```python
from build123d import *

# Parameters (mm, degrees)
BOSS_EXTRUDE1_DEPTH = 15
SKETCH2_R           = 1.7
SKETCH2_R_2         = 1.35
CUT_EXTRUDE1_DEPTH  = 59.066473529
CUT_EXTRUDE2_DEPTH  = 1


with BuildPart() as part:
    # Sketch1 → Boss-Extrude1 (new body)
    with BuildSketch(Plane.XY):
        with BuildLine():
            Line((0, 0), (35, 0))
            ThreePointArc((35, 0), (43.574008742, 1.66873563), (50.896306384, 6.431325448))
            ThreePointArc((50.896306384, 6.431325448), (52.409115124, 10), (50.896306384, 13.568674552))
            ThreePointArc((50.896306384, 13.568674552), (43.574008742, 18.33126437), (35, 20))
            Line((35, 20), (0, 20))
            Line((0, 20), (0, 17))
            Line((0, 17), (35.015119776, 17))
            ThreePointArc((35.015119776, 17), (42.445641677, 15.557658707), (48.796934125, 11.440124447))
            ThreePointArc((48.796934125, 11.440124447), (49.409115124, 10), (48.796934125, 8.559875553))
            ThreePointArc((48.796934125, 8.559875553), (42.445641677, 4.442341293), (35.015119776, 3))
            Line((35.015119776, 3), (0, 3))
            Line((0, 3), (0, 0))
        make_face()
    extrude(amount=BOSS_EXTRUDE1_DEPTH)

    # Sketch2 → Cut-Extrude1 (cut, through all)
    with BuildSketch(Plane(origin=(0, 20, 0), x_dir=(1, 0, 0), z_dir=(0, 1, 0))):
        with Locations(Location((5, -7.5, 0), (0, 0, 270))):
            Circle(SKETCH2_R)
        with Locations(Location((13.5, -7.5, 0), (0, 0, 270))):
            Circle(SKETCH2_R_2)
        with Locations(Location((31.5, -7.5, 0), (0, 0, 270))):
            Circle(SKETCH2_R_2)
    extrude(amount=-CUT_EXTRUDE1_DEPTH, mode=Mode.SUBTRACT)

    # Sketch3 → Cut-Extrude2 (cut)
    with BuildSketch(Plane.XZ):
        Polygon((5, 10.848631561), (2.1, 9.174315781), (2.1, 5.825684219), (5, 4.151368439), (7.9, 5.825684219), (7.9, 9.174315781), align=None)
    extrude(amount=-CUT_EXTRUDE2_DEPTH, mode=Mode.SUBTRACT)


solid = part.part
```
CAD build for the part. Positions are in the model's coordinates, mm. A direction names the side the tool comes from. Coordinates: 2 decimals unless noted, no trailing zeros. Order: outer loops, then holes, each group sorted by start corner. A loop starts at its lowest first (then second) coordinate and runs counter-clockwise, first axis right, second up. Notation, with made-up numbers: (42.5, 38) - (57.5, 38) arc R30 ccw to (57.5, 77) - close; hole circle Ø10 at (51.25, 25). An arc over 180 degrees is marked (long way). Use a Markdown table: item, result. Add a question column.
(1) Saw through at C-C (y = 2.5). Give the cut face in (x, z).
(2) Saw through at B-B (x = 23). Give the cut face in (y, z).
(3) Flat gauge pins, fed straight in: pin 1 (4.5 mm diameter, centred on x = 31.5, z = 7.5, fed in from +Y); pin 2 (1 mm diameter, centred on x = 42, z = 10, fed in from -Y); pin 3 (5 mm diameter, centred on y = 5, z = 13.5, fed in from +X); pin 4 (2.5 mm diameter, centred on x = 31.5, z = 7.5, fed in from -Y). Where does each tip first touch, or does it go through?
(4) Which spindle directions (+Z, -Z, +X, -X, +Y, -Y) get a long thin tool onto all of the face, cutting with end or side? Do faces 1 (the face through (3.53, 0.49, 5)), 2 (the face through (14.638, 18.521, 8.226)), 3 (the face through (18, 3, 7)). Say none if no direction does.
(5) Pull direction X, two halves, no side cores. Call faces 4 (the face through (7.9, 0.5, 7.5)), 5 (the face through (18, 20, 7)), 6 (the face through (42.347, 15.597, 7.395)): +X half, -X half, draft (parallel to the pull), parting line (faces both ways), or undercut.
(6) Saw through at A-A (x = 13.5). Give the cut face in (y, z), then the cut area to 3 significant figures.
(7) Saw through at D-D (z = 7.5). Count the separate pieces of the cut face and the enclosed holes in it, then the cut area to 3 significant figures.
(8) Drill centre lines: line 1 along Y through (x, z) = (25.5, 12.25); line 2 along X through (y, z) = (1.8, 7.5); line 3 along Y through (x, z) = (43, 13.75). Where is each one in solid material? Low to high. Write a range as [from, to].
Solved:
| question | item | result |
|---|---|---|
| 1 | outline | (0, 0) - (45.39, 0) - (45.39, 15) - (0, 15) - close; hole circle Ø3.4 at (5, 7.5); hole circle Ø2.7 at (13.5, 7.5); hole circle Ø2.7 at (31.5, 7.5) |
| 2 | outline | (0, 0) - (3, 0) - (3, 15) - (0, 15) - close; (17, 0) - (20, 0) - (20, 15) - (17, 15) - close |
| 3 | pin 1 | stops at y = 20 |
| 3 | pin 2 | stops at y = 0.94 |
| 3 | pin 3 | stops at x = 51.73 |
| 3 | pin 4 | passes through |
| 4 | face 1 | -Y |
| 4 | face 2 | +Y, -Y |
| 4 | face 3 | +Z, -Z, -X |
| 5 | face 4 | undercut |
| 5 | face 5 | draft |
| 5 | face 6 | -X half |
| 6 | outline | (0, 0) - (3, 0) - (3, 6.15) - (0, 6.15) - close; (0, 8.85) - (3, 8.85) - (3, 15) - (0, 15) - close; (17, 0) - (20, 0) - (20, 6.15) - (17, 6.15) - close; (17, 8.85) - (20, 8.85) - (20, 15) - (17, 15) - close |
| 6 | area | 73.8 mm² |
| 7 | separate pieces | 7 |
| 7 | enclosed holes | 0 |
| 7 | area | 270 mm² |
| 8 | line 1 | y = [0, 3], [17, 20] |
| 8 | line 2 | x = [0, 3.3], [6.7, 12.15], [14.85, 30.15], [32.85, 43.89] |
| 8 | line 3 | y = [1.45, 4.68], [15.32, 18.55] |
